Could you check a few things on this model? Use its own coordinates, in mm. Face numbers are marked on the shaded views. Coordinates: 2 decimals unless noted, no trailing zeros. Order: outer loops, then holes, each group sorted by start corner. A loop starts at its lowest first (then second) coordinate and runs counter-clockwise, first axis right, second up.
```python
from build123d import *

# Parameters (mm, degrees)
SKETCH1_R           = 1.42
BOSS_EXTRUDE1_DEPTH = 5
FILLET1_R           = 2


with BuildPart() as part:
    # Sketch1 → Boss-Extrude1 (new body)
    with BuildSketch(Plane(origin=(0, 0, 0), x_dir=(1, 0, 0), z_dir=(0, 1, 0))):
        with BuildLine():
            Line((-19.364916731, -5), (19.364916731, -5))
            ThreePointArc((19.364916731, -5), (0, 20), (-19.364916731, -5))
        make_face()
        with Locations((-5, 0)):
            Circle(SKETCH1_R, mode=Mode.SUBTRACT)
        with Locations((5, 0)):
            Circle(SKETCH1_R, mode=Mode.SUBTRACT)
    extrude(amount=BOSS_EXTRUDE1_DEPTH)

    # Sketch2 → Revolve1 (revolve)
    with BuildSketch(Plane.XY.offset(-11)):
        with BuildLine():
            Line((0, 5), (0, 40))
            ThreePointArc((0, 40), (-2.026770623, 39.21183201), (-2.988584094, 37.261467228))
            Line((-2.988584094, 37.261467228), (-5.811096745, 5))
            Line((-5.811096745, 5), (0, 5))
        make_face()
    revolve(axis=Axis((0, 5, -11), (0, 1, 0)))

    # Fillet1
    fillet1_edges = [part.edges().sort_by_distance(p)[0] for p in [
        (5.811096745, 5, -11),
    ]]
    fillet(fillet1_edges, radius=FILLET1_R)


solid = part.part
```
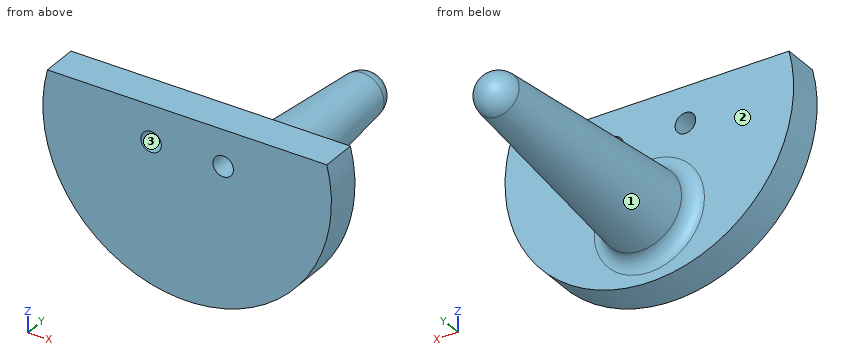
Item 1: Suppose I cut it at D-D (x = -8.5). List the corners of the cut face in (y, z) for me.
Item 2: Suppose I cut it at C-C (y = 33.5). List the corners of the cut face in (x, z) for me, and give its area (3 significant figures).
Item 3: Suppose I cut it at A-A (x = 0). List the corners of the cut face in (y, z) for me.
Item 4: Suppose I cut it at B-B (z = -11). List the corners of the cut face in (x, y) for me, and give its area (3 significant figures).
Item 5: Thinking about a two-plate mould opening in X: for the marked faces 1, 2 and 3, which applies, +X half, -X half, draft (parallel to the pull), parting line (faces both ways), or undercut?
Item 6: I need wall thicknesses on line 1 (X direction, y = 3.6, z = 0); line 2 (Z direction, x = 5, y = 3.3); line 3 (Y direction, x = -14.5, z = 4). Which ranges of each line are inside material? Lowest first, please.
Item 7: For pin 1 Ø1 at (x, y) = (-16, 6.5) entering from -Z; pin 2 Ø4.5 at (x, z) = (-5, 0) entering from +Y; pin 3 Ø10 at (x, y) = (1.5, 23) entering from +Z, each with a flat end and sliding along its axis, tell me the tip position at first contact or that it passes through.
Geometry results:
1. outline: (0, -18.1) - (5, -18.1) - (5, 5) - (0, 5) - close
2. outline: circle Ø6.64 at (0, -11)
2. area: 34.6 mm2
3. outline: (0, -20) - (5, -20) - (5, -18.64) arc R2 cw to (6.83, -16.65) - (37.26, -13.99) arc R3 ccw to (37.26, -8.01) - (6.83, -5.35) arc R2 cw to (5, -3.36) - (5, 5) - (0, 5) - close
4. outline: (-16.7, 0) - (16.7, 0) - (16.7, 5) - (7.64, 5) arc R2 cw to (5.65, 6.83) - (2.99, 37.26) arc R3 ccw to (-2.99, 37.26) - (-5.65, 6.83) arc R2 cw to (-7.64, 5) - (-16.7, 5) - close
4. area: 465 mm2
5. face 1: parting line
5. face 2: draft
5. face 3: undercut
6. line 1: x = -20 to -6.42, -3.58 to 3.58, 6.42 to 20
6. line 2: z = -19.36 to -1.42, 1.42 to 5
6. line 3: y = 0 to 5
7. pin 1: passes through
7. pin 2: stops at y = 5
7. pin 3: stops at z = -6.34
